Work out the finished part from the listing and answer in its coordinate system (mm). Face numbers are marked on the shaded views. A direction names the side the tool comes from. Coordinates: 2 decimals unless noted, no trailing zeros. Loops run counter-clockwise (first coordinate to the right, second up) from the corner with the lowest first, then second, coordinate; pieces in that order, holes last. Notation, with made-up numbers: (51.25, 85.25) - (70.25, 85.25) arc R12 ccw to (70.25, 90.25) - close; hole circle Ø9 at (11, 88.25). An arc over 180 degrees is marked (long way). Write each question's results on one line, items separated by ' | '. Start each with the question number.
Item 1: A tool of negligible diameter and unlimited length cuts with its end or side. For the marked faces 1 and 2, from which of +Z, -Z, +X, -X, +Y, -Y can it reach the whole face along a straight path? Write none if from no direction.
Item 2: Section A-A, the plane y = 26 is taken. Write down the section's boundary in (x, z).
Item 3: Section C-C, the plane x = -25 is taken. Write down the section's boundary in (y, z), plus the area to 3 significant figures.
Item 4: For a pull along X with two mould halves and no side action, classify the marked faces 3 and 4 as +X half, -X half, draft (parallel to the pull), parting line (faces both ways), or undercut.
Item 5: Each of these flat-tipped pins is pushed along its axis until it touches: pin 1 Ø5 at (x, y) = (17.5, 34.5) entering from -Z; pin 2 Ø17 at (x, z) = (3, -13.5) entering from -Y. Where does it stop, or does it pass through?
Item 6: Section B-B, the plane z = -43.5 is taken. Write down the section's boundary in (x, y).
Item 7: Consider probe 1 along Z at (x, y) = (19, 29.25); probe 2 along X at (y, z) = (28, -40); probe 3 along Y at (x, z) = (10.5, -3). Determine where each line is inside the solid, lowest interval first. Write a range as [from, to].
Autodesk Inventor part; units mm, degrees
ref_plane "YZ Plane" through (0, 0, 0) normal (1, 0, 0) x (0, 1, 0)
ref_plane "XZ Plane" through (0, 0, 0) normal (0, 1, 0) x (-1, 0, 0)
ref_plane "XY Plane" through (0, 0, 0) normal (0, 0, 1) x (1, 0, 0)
ref_plane "Plan de construction3" through (0, 20, 0) normal (0, 1, 0) x (1, 0, 0)
sketch "Esquisse7" plane through (0, 20, 0) normal (0, 1, 0) x (1, 0, 0)
  line L0 (-31.9796, 92.3061) -> (-31.9796, -36.6939)
  line L1 (28.0204, 92.3061) -> (-31.9796, 92.3061)
  line L2 (-31.9796, -36.6939) -> (28.0204, -36.6939)
  line L3 (28.0204, -36.6939) -> (28.0204, 92.3061)
  line L4 (28.0204, 92.3061) -> (-31.9796, 92.3061)
  line L5 (-31.9796, 92.3061) -> (-31.9796, -36.6939)
  line L6 (26.0204, 90.3061) -> (-29.9796, 90.3061)
  line L7 (26.0204, 90.3061) -> (26.0204, -34.6939)
  line L8 (-29.9796, 90.3061) -> (26.0204, 90.3061)
  line L9 (26.0204, 90.3061) -> (26.0204, -34.6939)
  line L10 (26.0204, -34.6939) -> (-29.9796, -34.6939)
  line L11 (-29.9796, -34.6939) -> (-29.9796, 90.3061)
  point P0 (0, 0)
  point P1 (6.0204, 92.3061)
extrude "Extrusion6" add sketch "Esquisse7" along normal blind 14
ref_plane "Plan de construction4" through (0, 34, 0) normal (0, 1, 0) x (1, 0, 0)
sketch "Esquisse8" plane through (0, 34, 0) normal (0, 1, 0) x (1, 0, 0)
  line L0 (-31.9796, 92.3061) -> (-31.9796, -36.6939)
  line L1 (28.0204, -36.6939) -> (28.0204, 92.3061)
  line L2 (-31.9796, -36.6939) -> (28.0204, -36.6939)
  line L3 (28.0204, -36.6939) -> (28.0204, 92.3061)
  line L4 (28.0204, 92.3061) -> (-31.9796, 92.3061)
  line L5 (-31.9796, 92.3061) -> (-31.9796, -36.6939)
  point P0 (0, 0)
extrude "Extrusion8" add sketch "Esquisse8" along normal blind 2
ref_plane "Plan de construction6" through (0, 36, 0) normal (0, 1, 0) x (1, 0, 0)
sketch "Esquisse9" plane through (0, 36, 0) normal (0, 1, 0) x (1, 0, 0)
  circle A0 centre (10.0204, -29.6939) radius 5
  line L0 (28.0204, -36.6939) -> (28.0204, 92.3061)
  line L1 (-31.9796, -36.6939) -> (28.0204, -36.6939)
  point P0 (0, 0)
  dimension "d75" = 10
  dimension "d76" = 18
  dimension "d77" = 7
extrude "Extrusion9" cut sketch "Esquisse9" against normal blind 3
ref_plane "Plan de construction5" through (0, 36, 0) normal (0, 1, 0) x (1, 0, 0)
sketch "Esquisse10" plane through (0, 36, 0) normal (0, 1, 0) x (1, 0, 0)
  circle A0 centre (23.0204, -30.6939) radius 2.5
  circle A1 centre (10.0204, -29.6939) radius 5
  line L0 (-31.9796, -36.6939) -> (28.0204, -36.6939)
  point P0 (0, 0)
  dimension "d80" = 13
  dimension "d81" = 5
  dimension "d82" = 6
extrude "Extrusion10" cut sketch "Esquisse10" against normal blind 3 contours A0
ref_plane "Plan de construction1" through (0, 18, 0) normal (0, 1, 0) x (1, 0, 0)
ref_plane "Plan de construction2" through (0, 20, 0) normal (0, 1, 0) x (1, 0, 0)
fillet "Congé6" radius 2 8 edges at (28.0204, 36, -27.8061) (28.0204, 28, -92.3061) (28.0204, 28, 36.6939) (-31.9796, 28, -92.3061) (-1.9796, 36, -92.3061) (-31.9796, 36, -27.8061) (-1.9796, 36, 36.6939) (-31.9796, 28, 36.6939)
fillet "Congé7" radius 1 1 edges at (20.5204, 36, 30.6939)
fillet "Congé8" radius 0.5 1 edges at (5.0204, 36, 29.6939)
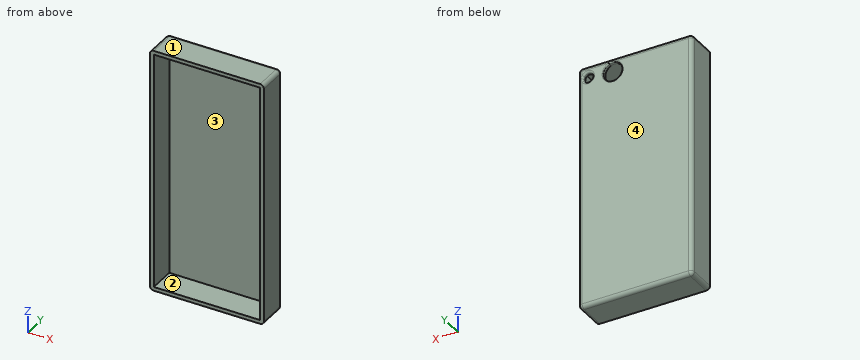
Answer key:
1) face 1: +Z, +X, -X, +Y, -Y | face 2: -Y
2) outline: (-31.98, -90.31) arc R2 ccw to (-29.98, -92.31) - (26.02, -92.31) arc R2 ccw to (28.02, -90.31) - (28.02, 34.69) arc R2 ccw to (26.02, 36.69) - (-29.98, 36.69) arc R2 ccw to (-31.98, 34.69) - close; hole (-29.98, -90.31) - (26.02, -90.31) - (26.02, 34.69) - (-29.98, 34.69) - close
3) outline: (20, -92.31) - (34, -92.31) arc R2 ccw to (36, -90.31) - (36, 34.69) arc R2 ccw to (34, 36.69) - (20, 36.69) - (20, 34.69) - (34, 34.69) - (34, -90.31) - (20, -90.31) - close | area: 312 mm^2
4) face 3: undercut | face 4: draft
5) pin 1: stops at z = -92.31 | pin 2: stops at y = 34
6) outline: (-31.98, 20) - (-29.98, 20) - (-29.98, 34) - (26.02, 34) - (26.02, 20) - (28.02, 20) - (28.02, 34) arc R2 ccw to (26.02, 36) - (-29.98, 36) arc R2 ccw to (-31.98, 34) - close
7) probe 1: z = [-92.31, -90.31], [34.69, 36.69] | probe 2: x = [-31.98, -29.98], [26.02, 28.02] | probe 3: y = [34, 36]
